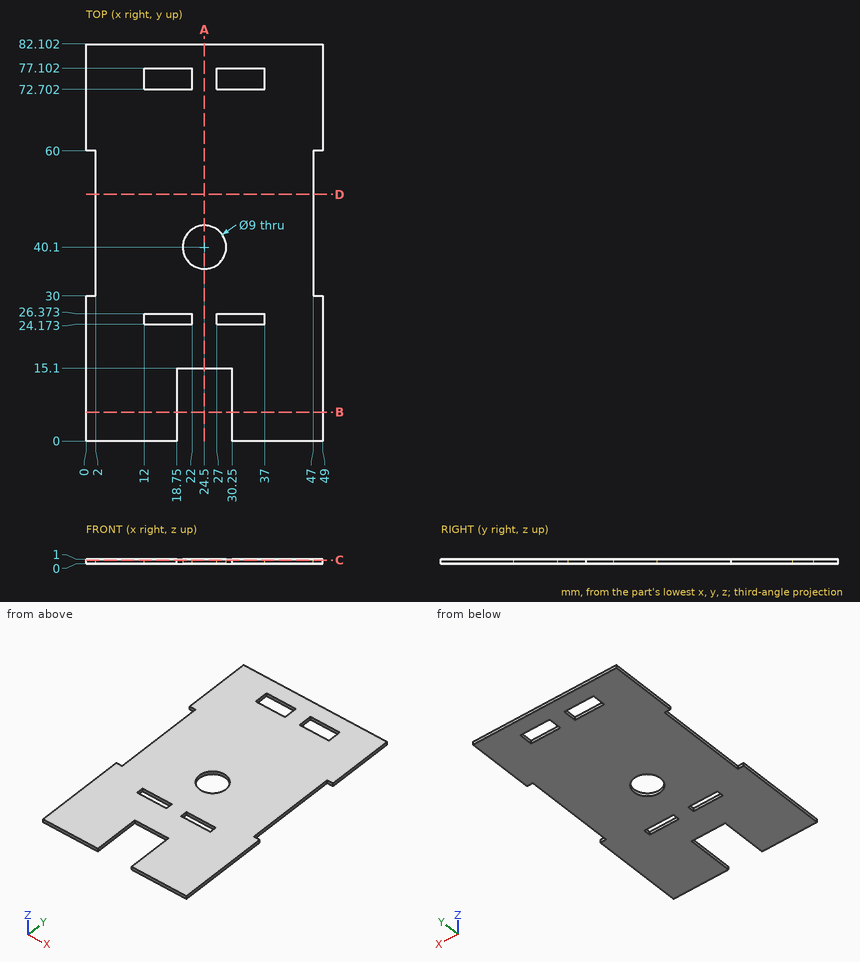
Print and shaded views of the part. All mm, measured from the part's lowest x, y and z. Round coordinates to 2 decimals unless told otherwise and drop trailing zeros. Write each loop counter-clockwise with the first axis right and the second up, starting at its lowest first coordinate (ties: lowest second). Pieces come first, ordered by that corner, then holes.
(1) Drop flat-ended pins along their axis: P1, Ø0.5, axis at y = 44.5, z = 0.5, coming from the +X side; P2, Ø5.5, axis at x = 24.5, y = 40.1, coming from the -Z side (3 decimals); P3, Ø12, axis at x = 17, y = 52.5, coming from the -Z side; P4, Ø0.5, axis at y = 41, z = 0.5, coming from the -X side. Give the stop position or say it passes through.
(2) Probe line 1 along Y through (x, z) = (12.5, 0.85); line 2 along Y through (x, z) = (24.5, 0.85); line 3 along Y through (x, z) = (28, 0.6) (1 decimal). List the from-to ranges inside material, lowest first.
(3) Slice it at D-D, the plane y = 51. Write the cut outline in (x, z).
(4) Slice it at A-A, the plane x = 24.5. Write the cut outline in (y, z).
(5) Slice it at C-C, the plane z = 0.8. Count the separate pieces of the cut face and the enclosed holes in it, and give its area (3 significant figures).
(6) Slice it at B-B, the plane y = 6. Write the cut outline in (x, z).
From the geometry:
1. P1: stops at x = 47
1. P2: passes through
1. P3: stops at z = 0
1. P4: stops at x = 2
2. line 1: y = 0 to 24.17, 26.37 to 72.7, 77.1 to 82.1
2. line 2: y = 15.1 to 35.6, 44.6 to 82.1
2. line 3: y = 15.1 to 24.2, 26.4 to 37.3, 42.9 to 72.7, 77.1 to 82.1
3. outline: (2, 0) - (47, 0) - (47, 1) - (2, 1) - close
4. outline: (15.1, 0) - (35.6, 0) - (35.6, 1) - (15.1, 1) - close; (44.6, 0) - (82.1, 0) - (82.1, 1) - (44.6, 1) - close
5. separate pieces: 1
5. enclosed holes: 5
5. area: 3,530 mm2
6. outline: (0, 0) - (18.75, 0) - (18.75, 1) - (0, 1) - close; (30.25, 0) - (49, 0) - (49, 1) - (30.25, 1) - close
